from build123d import *

# Parameters (mm, degrees)
F0_R     = 9.525
F1_DEPTH = 25.4
F3_R     = 4.7625
F4_DEPTH = 25.401
F2_W     = 9.525
F2_H     = 9.525
F5_DEPTH = 11.0998
F7_DEPTH = 9.525


with BuildPart() as f1:
    # F0 (on Front) → F1 (new body)
    with BuildSketch(Plane.XZ):
        Circle(F0_R)
    extrude(amount=F1_DEPTH)

    # F3 (on Front) → F4 (cut, through all)
    with BuildSketch(Plane.XZ):
        Circle(F3_R)
    extrude(amount=F4_DEPTH, mode=Mode.SUBTRACT)

    # F2 (on Front) → F5 (cut)
    with BuildSketch(Plane.XZ):
        Rectangle(F2_W, F2_H)
    extrude(amount=F5_DEPTH, mode=Mode.SUBTRACT)

    # F6 (on face) → F7 (cut)
    with BuildSketch(Plane.XZ.offset(25.4)):
        Polygon((3.65125, 6.324151), (-3.65125, 6.324151), (-7.3025, 0), (-3.65125, -6.324151), (3.65125, -6.324151), (7.3025, 0), align=None)
    extrude(amount=-F7_DEPTH, mode=Mode.SUBTRACT)


solid = f1.part
Source: CAD feature listing. Evaluate the final solid. Frame: model axes, mm. A direction names the side the tool comes from. Give positions to 0.01 mm unless a question says otherwise; leave off trailing zeros. Write each loop counter-clockwise with the first axis right and the second up, starting at its lowest first coordinate (ties: lowest second). Pieces come first, ordered by that corner, then holes. Notation, with made-up numbers: (-35.5, 17.5) -> (-9.5, 17.5) arc R33 cw to (-9.5, 48.5) -> close; hole circle Ø7 at (42, 63). An arc over 180 degrees is marked (long way). Return JSON: item names as keys, results as strings. Group by question number.
1. Pin query (flat end, axial travel): pin 1 Ø2 at (y, z) = (-11.5, -1.5) entering from -X; pin 2 Ø10.5 at (x, y) = (1.5, -4) entering from +Z (3 decimals); pin 3 Ø1.5 at (y, z) = (-5, -5.5) entering from -X; pin 4 Ø4 at (x, z) = (-2, -2) entering from +Y. Return the tip coordinate at first contact, or that it passes through.
2. Access query for faces 1 (the face through (-3.78, -13.45, -2.9)), 2 (the face through (-4, -11.1, 4)), 3 (the face through (5, -15.875, 0)). Directions: +Z, -Z, +X, -X, +Y, -Y. A direction counts if a zero-diameter tool reaches every point of the face in a straight line with its end or side. Return the directions, or none.
3. Section D-D, the plane x = -5.5. Output: boundary loops of the cut face in (y, z) (3 decimals).
4. Section B-B, the plane z = 2.5. Output: boundary loops of the cut face in (x, y) (1 decimal).
5. Mould query, pull axis Z, two halves, no side actions, for faces 4 (the face through (4, -11.1, -4)), 5 (the face through (0, 0, -6)), 6 (the face through (0, -21, -6.324)), 7 (the face through (-7.559, -12.522, -5.796)). Classes: +Z half, -Z half, draft (parallel to the pull), parting line (faces both ways), or undercut.
6. Material intervals for line 1 (Z direction, x = 0, y = -14.5) (1 decimal); line 2 (Z direction, x = -3.75, y = -15); line 3 (Y direction, x = -1.5, z = 5.25) (3 decimals), sorted ascending. Write a range as from..to.
Determined:
{
 "1": {"pin 1": "stops at x = -9.51", "pin 2": "stops at z = 9.525", "pin 3": "stops at x = -8.26", "pin 4": "stops at y = -11.1"},
 "2": {"face 1": "+Y, -Y", "face 2": "+Y", "face 3": "-Y"},
 "3": {"outline": "(-25.4, -7.777) -> (0, -7.777) -> (0, 7.777) -> (-25.4, 7.777) -> (-25.4, 3.122) -> (-15.875, 3.122) -> (-15.875, -3.122) -> (-25.4, -3.122) -> close"},
 "4": {"outline": "(-9.2, -25.4) -> (-5.9, -25.4) -> (-5.9, -15.9) -> (-4.1, -15.9) -> (-4.1, -11.1) -> (-4.8, -11.1) -> (-4.8, 0) -> (-9.2, 0) -> close; (4.1, -15.9) -> (5.9, -15.9) -> (5.9, -25.4) -> (9.2, -25.4) -> (9.2, 0) -> (4.8, 0) -> (4.8, -11.1) -> (4.1, -11.1) -> close"},
 "5": {"face 4": "undercut", "face 5": "draft", "face 6": "undercut", "face 7": "parting line"},
 "6": {"line 1": "z = -9.5..-4.8, 4.8..9.5", "line 2": "z = -8.76..-2.94, 2.94..8.76", "line 3": "y = -15.875..0"}
}
